The listing builds one solid part. Answer for the finished solid, in the listing's coordinates (mm). A direction names the side the tool comes from. Give positions to 0.01 mm unless a question says otherwise; leave off trailing zeros. Order: outer loops, then holes, each group sorted by start corner. A loop starts at its lowest first (then second) coordinate and runs counter-clockwise, first axis right, second up. Notation, with made-up numbers: (5.25, 80) - (55.25, 80) arc R21 cw to (55.25, 95) - close; hole circle Ø9 at (-34.75, 5). An arc over 180 degrees is marked (long way). Answer as a JSON object with one key per item and string values. Group by question number.
Q1. For faces 4 (the face through (0, 0, 2)), 5 (the face through (0, -2.794, 0)), 6 (the face through (2.769, 1.878, -5.323)), determine the directions among +Z, -Z, +X, -X, +Y, -Y from which every point of the face is accessible in a straight line to the end or side of a thin tool.
Q2. A cutting plane is placed at C-C, the plane y = 7.25. Give the vertices of the cut face in (x, z).
Q3. A cutting plane is placed at A-A, the plane x = 0. Give the vertices of the cut face in (y, z).
Q4. Consider line 1 (Y direction, x = 3.25, z = 5); line 2 (X direction, y = 4.75, z = -5); line 3 (X direction, y = 4, z = -1.5). Determine where each line is inside the solid, lowest interval first.
Q5. A cutting plane is placed at D-D, the plane z = 3.5. Give the vertices of the cut face in (x, y), and give its area (3 significant figures).
Q6. A cutting plane is placed at B-B, the plane z = -4.75. Give the vertices of the cut face in (x, y), and give its area (3 significant figures).
Q7. The mould has two halves that part along X. Classify faces 1 (the face through (-0.56, 3.77, -2.96)), 2 (the face through (6.364, -1.893, 0.836)), 3 (the face through (0.1, 3.5, 0)): released by +X, released by -X, zero draft, split by the parting line, or undercut.
Q8. Given pin 1 (3 mm diameter, centred on x = 0, y = 6.29, fed in from +Z); pin 2 (3 mm diameter, centred on y = 7, z = 0, fed in from +X); pin 3 (1 mm diameter, centred on x = -2, z = -2, fed in from +Y); pin 4 (6.5 mm diameter, centred on x = 2.5, z = 4, fed in from +Y), each flat-ended and moving along its own axis, determine where each tip first touches the part or whether it passes through.
from build123d import *
from build123d.topology import SkipClean

# Parameters (mm, degrees)
REVOLVE1_ANGLE = 180
SKETCH2_R      = 6
EXTRUDE1_DEPTH = 1.016
SKETCH3_R      = 6.419039945
EXTRUDE2_DEPTH = 1.778
SKETCH4_R      = 2.584873193
EXTRUDE3_DEPTH = 16.281774039


with BuildPart() as part:
    # Sketch1 → Revolve1 (revolve)
    with BuildSketch(Plane.XY):
        with BuildLine():
            Line((-6, 0), (-6, 6.293269303))
            ThreePointArc((-6, 6.293269303), (-4.242640687, 10.535909991), (0, 12.293269303))
            Line((0, 12.293269303), (0, 0))
            Line((0, 0), (-6, 0))
        make_face()
    revolve(axis=Axis((0, 12.293269303, 0), (0, -1, 0)), revolution_arc=REVOLVE1_ANGLE)

    # Sketch2 → Extrude1 (add)
    with BuildSketch(Plane.XZ):
        Circle(SKETCH2_R)
    extrude(amount=EXTRUDE1_DEPTH)

    # Sketch3 → Extrude2 (add)
    with BuildSketch(Plane.XZ.offset(1.016)):
        with Locations(Location((0, 0, 0), (0, 0, 270))):
            Circle(SKETCH3_R)
    extrude(amount=EXTRUDE2_DEPTH)

    # Sketch4 → Extrude3 (cut, through all)
    with SkipClean():  # the faces are left unmerged after this step: merging them gives an invalid solid
        with BuildSketch(Plane.XY):
            with Locations((0, 6.293269303)):
                Circle(SKETCH4_R)
        extrude(amount=-EXTRUDE3_DEPTH, mode=Mode.SUBTRACT)


solid = part.part
Reply:
{
 "1": {"face 4": "+Z, +X, -X, +Y", "face 5": "+Z, -Z, +X, -X, -Y", "face 6": "+Y"},
 "2": {"outline": "(-5.92, 0) arc R5.92 ccw to (-2.4, -5.41) - (-2.4, 0) - close; (2.4, -5.41) arc R5.92 ccw to (5.92, 0) - (2.4, 0) - close"},
 "3": {"outline": "(-2.79, -6.42) - (-1.02, -6.42) - (-1.02, -6) - (3.71, -6) - (3.71, 0) - (0, 0) - (0, 6) - (-1.02, 6) - (-1.02, 6.42) - (-2.79, 6.42) - close; (8.88, -5.41) arc R6 ccw to (12.29, 0) - (8.88, 0) - close"},
 "4": {"line 1": "y = -2.79 to 0", "line 2": "x = -3.32 to -2.07, 2.07 to 3.32", "line 3": "x = -5.81 to -1.19, 1.19 to 5.81"},
 "5": {"outline": "(-5.38, -2.79) - (5.38, -2.79) - (5.38, -1.02) - (4.87, -1.02) - (4.87, 0) - (-4.87, 0) - (-4.87, -1.02) - (-5.38, -1.02) - close", "area": "29.0 mm^2"},
 "6": {"outline": "(-4.32, -2.79) - (4.32, -2.79) - (4.32, -1.02) - (3.67, -1.02) - (3.67, 6.29) arc R3.67 ccw to (-3.67, 6.29) - (-3.67, -1.02) - (-4.32, -1.02) - close; hole circle Ø5.17 at (0, 6.29)", "area": "69.1 mm^2"},
 "7": {"face 1": "undercut", "face 2": "split by the parting line", "face 3": "zero draft"},
 "8": {"pin 1": "passes through", "pin 2": "stops at x = 6", "pin 3": "stops at y = 11.82", "pin 4": "stops at y = 0"}
}
